Geometry: final body of the model. Coordinates: model frame, mm. A direction names the side the tool comes from. Round coordinates to 2 decimals unless told otherwise and drop trailing zeros. Loops run counter-clockwise (first coordinate to the right, second up) from the corner with the lowest first, then second, coordinate; pieces in that order, holes last. Notation, with made-up numbers: (24, 52) - (34, 52) arc R17 ccw to (34, 60) - close; hole circle Ø10 at (-12, -11). An arc over 180 degrees is marked (long way). Answer as a JSON object with one key per item and string values. Group by question number.
Item 1: Section B-B (x = 226.5). Return the cut outline in (y, z).
Item 2: Draft query along X for faces 6 (the face through (125, 79, 82.5)), 7 (the face through (252, 153, 39)), 8 (the face through (128, 79, 6.3)), 9 (the face through (128, 2, 3)). Return one class per face: released by +X, released by -X, zero draft, split by the parting line, or undercut.
Item 3: Reachability of faces 1 (the face through (-5, 134.5, 22)), 2 (the face through (2, 76, 3)), 3 (the face through (-5, 20.5, 22)), 4 (the face through (251, 1, 39)), 5 (the face through (125, 0, 38)) from +Z, -Z, +X, -X, +Y, -Y: full face, straight path, thin tool, end or side. Return the list, or none.
Item 4: Section C-C (z = 66). Return the cut outline in (x, y).
Item 5: Line query: line 1 (X direction, y = 135, z = 5); line 2 (Y direction, x = 152.5, z = 4); line 3 (Z direction, x = 224, y = 16.5). Output: solid intervals per line, ascending.
Item 6: Section D-D (y = 79). Return the cut outline in (x, z).
Item 7: First-contact query: pin 1 (8 mm diameter, centred on x = 107, y = 76.5, fed in from -Z); pin 2 (14 mm diameter, centred on x = -8, y = 49.5, fed in from +Z); pin 3 (2 mm diameter, centred on y = 91, z = 57.5, fed in from -X). Flat tips, straight axial feed; report the tip coordinate or a pass-through.
Item 8: Section A-A (y = 10). Return the cut outline in (x, z), plus the area to 3 significant figures.
```python
from build123d import *

# Parameters (mm, degrees)
SKETCH1_W           = 253
SKETCH1_H           = 155
BOSS_EXTRUDE1_DEPTH = 82.5
FILLET1_R           = 5
CUT_EXTRUDE1_DEPTH  = 6.3
SKETCH5_W           = 45
SKETCH5_H           = 114
BOSS_EXTRUDE2_DEPTH = 12.7
FILLET2_R           = 3


with BuildPart() as part:
    # Sketch1 → Boss-Extrude1 (new body)
    with BuildSketch(Plane.XY):
        with Locations((126.5, 77.5)):
            Rectangle(SKETCH1_W, SKETCH1_H)
    extrude(amount=BOSS_EXTRUDE1_DEPTH)

    # Fillet1
    fillet1_edges = [part.edges().sort_by_distance(p)[0] for p in [
        (126.5, 155, 82.5),
        (0, 77.5, 82.5),
        (126.5, 0, 82.5),
        (253, 77.5, 82.5),
        (0, 0, 41.25),
        (0, 155, 41.25),
        (253, 155, 41.25),
        (253, 0, 41.25),
    ]]
    fillet(fillet1_edges, radius=FILLET1_R)

    # Sketch2 → Cut-Extrude1 (cut)
    with BuildSketch(Plane(origin=(0, 0, 0), x_dir=(-1, 0, 0), z_dir=(0, 0, -1))):
        with BuildLine():
            Line((-2, 5), (-2, 150))
            ThreePointArc((-2, 150), (-2.878679656, 152.121320344), (-5, 153))
            Line((-5, 153), (-248, 153))
            ThreePointArc((-248, 153), (-250.121320344, 152.121320344), (-251, 150))
            Line((-251, 150), (-251, 5))
            ThreePointArc((-251, 5), (-250.121320344, 2.878679656), (-248, 2))
            Line((-248, 2), (-5, 2))
            ThreePointArc((-5, 2), (-2.878679656, 2.878679656), (-2, 5))
        make_face()
    extrude(amount=-CUT_EXTRUDE1_DEPTH, mode=Mode.SUBTRACT)

    # Sketch5 → Boss-Extrude2 (add)
    with BuildSketch(Plane.ZY):
        with Locations((22.5, 77.5)):
            Rectangle(SKETCH5_W, SKETCH5_H)
    extrude(amount=BOSS_EXTRUDE2_DEPTH)

    # Fillet2
    fillet2_edges = [part.edges().sort_by_distance(p)[0] for p in [
        (-12.7, 134.5, 22.5),
        (-12.7, 20.5, 22.5),
    ]]
    fillet(fillet2_edges, radius=FILLET2_R)


solid = part.part
```
Values:
{
 "1": {"outline": "(0, 0) - (2, 0) - (2, 6.3) - (153, 6.3) - (153, 0) - (155, 0) - (155, 77.5) arc R5 ccw to (150, 82.5) - (5, 82.5) arc R5 ccw to (0, 77.5) - close"},
 "2": {"face 6": "zero draft", "face 7": "released by +X", "face 8": "undercut", "face 9": "undercut"},
 "3": {"face 1": "+Z, -Z, -X, +Y", "face 2": "-Z", "face 3": "+Z, -Z, -X, -Y", "face 4": "+Z, -Z, +X, -Y", "face 5": "+Z, -Z, +X, -X, -Y"},
 "4": {"outline": "(0, 5) arc R5 ccw to (5, 0) - (248, 0) arc R5 ccw to (253, 5) - (253, 150) arc R5 ccw to (248, 155) - (5, 155) arc R5 ccw to (0, 150) - close"},
 "5": {"line 1": "x = 0 to 2, 251 to 253", "line 2": "y = 0 to 2, 153 to 155", "line 3": "z = 6.3 to 82.5"},
 "6": {"outline": "(-12.7, 0) - (2, 0) - (2, 6.3) - (251, 6.3) - (251, 0) - (253, 0) - (253, 77.5) arc R5 ccw to (248, 82.5) - (5, 82.5) arc R5 ccw to (0, 77.5) - (0, 45) - (-12.7, 45) - close"},
 "7": {"pin 1": "stops at z = 6.3", "pin 2": "stops at z = 45", "pin 3": "stops at x = 0"},
 "8": {"outline": "(0, 0) - (2, 0) - (2, 6.3) - (251, 6.3) - (251, 0) - (253, 0) - (253, 77.5) arc R5 ccw to (248, 82.5) - (5, 82.5) arc R5 ccw to (0, 77.5) - close", "area": "19,300 mm^2"}
}
